```python
from build123d import *

# Parameters (mm, degrees)
SKETCH1_W           = 24
SKETCH1_H           = 12
SKETCH1_R           = 1.2
SKETCH1_R_2         = 5
BOSS_EXTRUDE1_DEPTH = 1.5


with BuildPart() as part:
    # Sketch1 → Boss-Extrude1 (new body)
    with BuildSketch(Plane.XY):
        with Locations((12, 6)):
            Rectangle(SKETCH1_W, SKETCH1_H)
        with Locations((2, 10)):
            Circle(SKETCH1_R, mode=Mode.SUBTRACT)
        with Locations(Location((22, 10, 0), (0, 0, 180))):
            Circle(SKETCH1_R, mode=Mode.SUBTRACT)
        with Locations((22, 2)):
            Circle(SKETCH1_R, mode=Mode.SUBTRACT)
        with Locations(Location((2, 2, 0), (0, 0, 180))):
            Circle(SKETCH1_R, mode=Mode.SUBTRACT)
        with Locations((12, 6)):
            Circle(SKETCH1_R_2, mode=Mode.SUBTRACT)
    extrude(amount=BOSS_EXTRUDE1_DEPTH)


solid = part.part
```
Verification items for the finished model (mm, model axes). Coordinates: 2 decimals unless noted, no trailing zeros. Loops run counter-clockwise (first coordinate to the right, second up) from the corner with the lowest first, then second, coordinate; pieces in that order, holes last. Notation, with made-up numbers: (-33.5, -27) - (-22.5, -27) arc R33 cw to (-22.5, 11) - close; hole circle Ø9 at (21.5, 24.25). An arc over 180 degrees is marked (long way). Answer as a JSON object with one key per item and string values.
(1) Cross-section at A-A, the plane x = 12. Record the boundary of the cut face in (y, z), then the cut area to 3 significant figures.
Response:
{"outline": "(0, 0) - (1, 0) - (1, 1.5) - (0, 1.5) - close; (11, 0) - (12, 0) - (12, 1.5) - (11, 1.5) - close", "area": "3.00 mm²"}
(2) Cross-section at D-D, the plane y = 6. Record the boundary of the cut face in (x, z), then the cut area to 3 significant figures.
Response:
{"outline": "(0, 0) - (7, 0) - (7, 1.5) - (0, 1.5) - close; (17, 0) - (24, 0) - (24, 1.5) - (17, 1.5) - close", "area": "21.0 mm²"}
(3) Mould release check, pull along Y, two halves, no side actions. Record for faces 1 (the flat face through (24, 6, 1)), 2 (the flat face through (12, 0, 1)), 3 (the cylindrical face through (22.95, 10.73, 0.74)): pulls with the +Y half, pulls with the -Y half, needs draft (parallel to the pull), parting line crosses it, or undercut.
Response:
{"face 1": "needs draft", "face 2": "pulls with the -Y half", "face 3": "undercut"}
(4) Cross-section at C-C, the plane x = 2. Record the boundary of the cut face in (y, z), then the cut area to 3 significant figures.
Response:
{"outline": "(0, 0) - (0.8, 0) - (0.8, 1.5) - (0, 1.5) - close; (3.2, 0) - (8.8, 0) - (8.8, 1.5) - (3.2, 1.5) - close; (11.2, 0) - (12, 0) - (12, 1.5) - (11.2, 1.5) - close", "area": "10.8 mm²"}
(5) Cross-section at B-B, the plane z = 1.2. Record the boundary of the cut face in (x, y), then the cut area to 3 significant figures.
Response:
{"outline": "(0, 0) - (24, 0) - (24, 12) - (0, 12) - close; hole circle Ø2.4 at (2, 2); hole circle Ø2.4 at (2, 10); hole circle Ø10 at (12, 6); hole circle Ø2.4 at (22, 2); hole circle Ø2.4 at (22, 10)", "area": "191 mm²"}
(6) Scan lines: line 1 along Y through (x, z) = (22, 0.95); line 2 along X through (y, z) = (2.5, 1.35); line 3 along Y through (x, z) = (21.5, 0.35). Record each from-to range of solid material in increasing order.
Response:
{"line 1": "y = 0 to 0.8, 3.2 to 8.8, 11.2 to 12", "line 2": "x = 0 to 0.91, 3.09 to 8.43, 15.57 to 20.91, 23.09 to 24", "line 3": "y = 0 to 0.91, 3.09 to 8.91, 11.09 to 12"}
